Source: three-view drawing plus pictorial views. Frame: mm from the lowest corner of the part. A direction names the side the tool comes from. Give positions to 0.01 mm unless a question says otherwise; leave off trailing zeros. Loops run counter-clockwise (first coordinate to the right, second up) from the corner with the lowest first, then second, coordinate; pieces in that order, holes last. Notation, with made-up numbers: (-26.5, 28) - (9.5, 28) arc R26 cw to (9.5, 48) - close; hole circle Ø10 at (40, 23.5). An arc over 180 degrees is marked (long way). Answer as a JSON object with one key per item and string values. Group by question number.
(1) Pin query (flat end, axial travel): P1, Ø22.5, axis at x = 72, y = 53, coming from the -Z side; P2, Ø23, axis at x = 66, z = 24, coming from the +Y side. Return the tip coordinate at first contact, or that it passes through.
(2) Access query for the marked faces 5, 6 and 7. Directions: +Z, -Z, +X, -X, +Y, -Y. A direction counts if a zero-diameter tool reaches every point of the face in a straight line with its end or side. Return the directions, or none.
(3) Material intervals for L1, parallel to X at y = 1, z = 64; L2, parallel to Z at x = 37.5, y = 49.5; L3, parallel to X at y = 21, z = 76.5, sorted ascending.
(4) Section query B-B (z = 64). Return loops of the section in (x, y), plus the area to 3 significant figures.
(5) Section query A-A (x = 41). Return loops of the section in (y, z), plus the area to 3 significant figures.
(6) Mould query, pull axis Z, two halves, no side actions, for the marked faces 1, 2, 3 and 4. Classes: +Z half, -Z half, draft (parallel to the pull), parting line (faces both ways), or undercut.
(7) Section query D-D (x = 65). Return loops of the section in (y, z).
(8) Section query C-C (z = 40). Return loops of the section in (x, y).
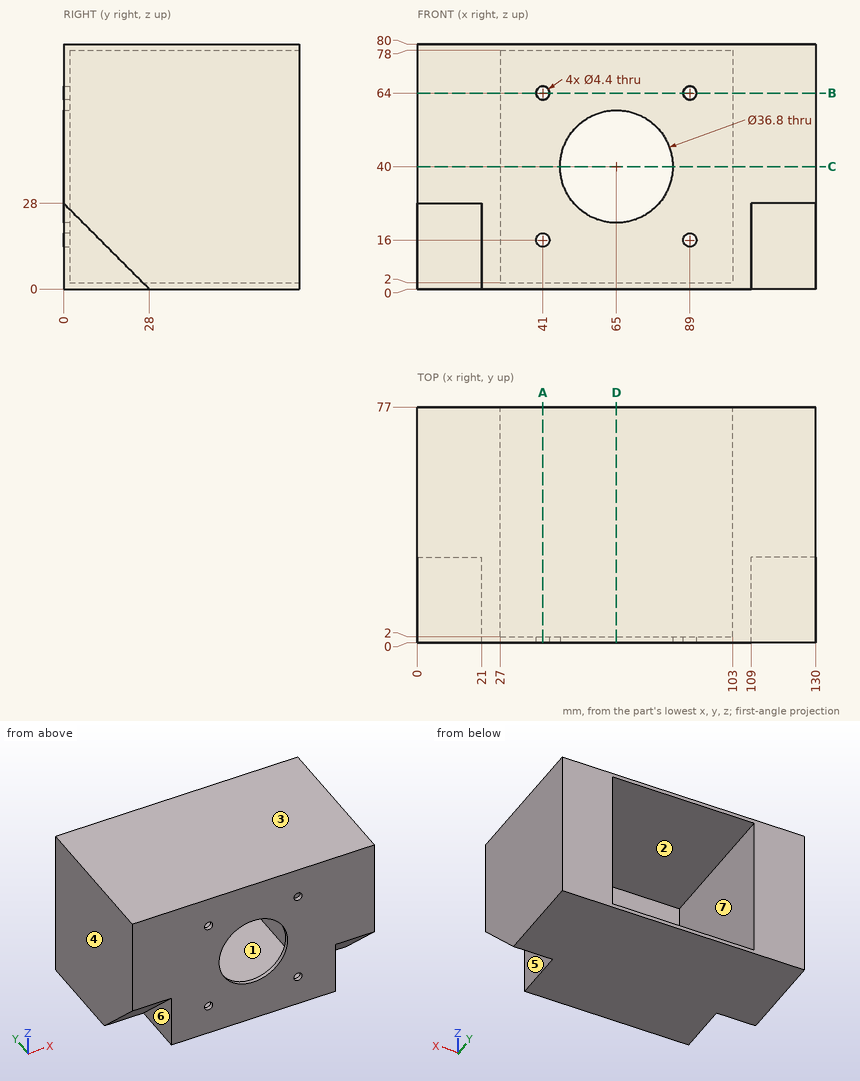
Recorded:
{
 "1": {"P1": "stops at z = 0", "P2": "stops at y = 2"},
 "2": {"face 5": "-Z, +X, -Y", "face 6": "-Z, -X, -Y", "face 7": "+Y"},
 "3": {"L1": "x = 0 to 38.8, 43.2 to 86.8, 91.2 to 130", "L2": "z = 0 to 2, 78 to 80", "L3": "x = 0 to 27, 103 to 130"},
 "4": {"outline": "(0, 0) - (38.8, 0) - (38.8, 2) - (27, 2) - (27, 77) - (0, 77) - close; (43.2, 0) - (86.8, 0) - (86.8, 2) - (43.2, 2) - close; (91.2, 0) - (130, 0) - (130, 77) - (103, 77) - (103, 2) - (91.2, 2) - close", "area": "4,290 mm^2"},
 "5": {"outline": "(0, 0) - (77, 0) - (77, 2) - (2, 2) - (2, 13.8) - (0, 13.8) - close; (0, 18.2) - (2, 18.2) - (2, 61.8) - (0, 61.8) - close; (0, 66.2) - (2, 66.2) - (2, 78) - (77, 78) - (77, 80) - (0, 80) - close", "area": "442 mm^2"},
 "6": {"face 1": "undercut", "face 2": "undercut", "face 3": "+Z half", "face 4": "draft"},
 "7": {"outline": "(0, 0) - (77, 0) - (77, 2) - (2, 2) - (2, 21.6) - (0, 21.6) - close; (0, 58.4) - (2, 58.4) - (2, 78) - (77, 78) - (77, 80) - (0, 80) - close"},
 "8": {"outline": "(0, 0) - (46.6, 0) - (46.6, 2) - (27, 2) - (27, 77) - (0, 77) - close; (83.4, 0) - (130, 0) - (130, 77) - (103, 77) - (103, 2) - (83.4, 2) - close"}
}
